from build123d import *

# Parameters (mm, degrees)
SKETCH1_W           = 150.5
SKETCH1_H           = 50
BOSS_EXTRUDE1_DEPTH = 3
SKETCH2_R           = 1.5
SKETCH2_R_2         = 1.25
CUT_EXTRUDE1_DEPTH  = 4
SKETCH4_W           = 74
SKETCH4_H           = 3.5
BOSS_EXTRUDE2_DEPTH = 3
SKETCH5_R           = 1.5
CUT_EXTRUDE3_DEPTH  = 4
SKETCH6_W           = 76.5
SKETCH6_H           = 3
SKETCH6_W_2         = 8
SKETCH6_W_3         = 2
SKETCH6_H_2         = 7
SKETCH6_W_4         = 4
SKETCH6_W_5         = 3
SKETCH6_H_3         = 18
SKETCH6_W_6         = 10
BOSS_EXTRUDE3_DEPTH = 18
SKETCH8_W           = 10
SKETCH8_H           = 3
SKETCH8_H_2         = 2
SKETCH8_W_2         = 42
SKETCH8_W_3         = 3
SKETCH8_H_3         = 15
BOSS_EXTRUDE4_DEPTH = 3
CUT_EXTRUDE4_REACH  = 55.5
SKETCH9_W           = 20
SKETCH9_H           = 10
CUT_EXTRUDE5_REACH  = 152.5
SKETCH10_R          = 1.25
SKETCH11_R          = 1.25
CUT_EXTRUDE6_DEPTH  = 54.5
SKETCH12_R          = 1.25
CUT_EXTRUDE7_DEPTH  = 58
SKETCH13_W          = 10
SKETCH13_H          = 1.5
CUT_EXTRUDE8_DEPTH  = 1.5


with BuildPart() as part:
    # Sketch1 → Boss-Extrude1 (new body)
    with BuildSketch(Plane(origin=(0, 0, 0), x_dir=(1, 0, 0), z_dir=(0, 1, 0))):
        with Locations((-39.87052506, -3.090692124)):
            Rectangle(SKETCH1_W, SKETCH1_H)
    extrude(amount=BOSS_EXTRUDE1_DEPTH)

    # Sketch2 → Cut-Extrude1 (cut, through all)
    with BuildSketch(Plane(origin=(0, 3, 0), x_dir=(1, 0, 0), z_dir=(0, 1, 0))):
        with Locations((-65.12052506, 12.159307876)):
            Circle(SKETCH2_R)
        with Locations((-65.12052506, -18.340692124)):
            Circle(SKETCH2_R)
        with Locations((-34.62052506, -18.340692124)):
            Circle(SKETCH2_R)
        with Locations((-34.62052506, 12.159307876)):
            Circle(SKETCH2_R)
        with Locations((17.87947494, -16.590692124)):
            Circle(SKETCH2_R)
        with Locations((17.87947494, 10.409307876)):
            Circle(SKETCH2_R)
        with Locations((-111.62052506, -19.090692124)):
            Circle(SKETCH2_R)
        with Locations((-111.62052506, 12.909307876)):
            Circle(SKETCH2_R)
        with Locations((-87.62052506, 11.909307876)):
            Circle(SKETCH2_R_2)
        with Locations((-87.62052506, -18.090692124)):
            Circle(SKETCH2_R_2)
        with Locations((-51.62052506, 12.909307876)):
            Circle(SKETCH2_R)
        with Locations((-51.62052506, -19.090692124)):
            Circle(SKETCH2_R)
    extrude(amount=-CUT_EXTRUDE1_DEPTH, mode=Mode.SUBTRACT)

    # Sketch4 → Boss-Extrude2 (add)
    with BuildSketch(Plane(origin=(0, 3, 0), x_dir=(1, 0, 0), z_dir=(0, 1, 0))):
        with Locations((-1.62052506, -29.840692124)):
            Rectangle(SKETCH4_W, SKETCH4_H)
        with Locations((-1.62052506, 23.659307876)):
            Rectangle(SKETCH4_W, SKETCH4_H)
    extrude(amount=-BOSS_EXTRUDE2_DEPTH)

    # Sketch5 → Cut-Extrude3 (cut, through all)
    with BuildSketch(Plane(origin=(0, 3, 0), x_dir=(1, 0, 0), z_dir=(0, 1, 0))):
        with Locations((-34.12052506, 19.409307876)):
            Circle(SKETCH5_R)
        with Locations((-34.12052506, -25.590692124)):
            Circle(SKETCH5_R)
        with Locations((10.87947494, 19.409307876)):
            Circle(SKETCH5_R)
        with Locations((10.87947494, -25.590692124)):
            Circle(SKETCH5_R)
    extrude(amount=-CUT_EXTRUDE3_DEPTH, mode=Mode.SUBTRACT)

    # Sketch6 → Boss-Extrude3 (add)
    with BuildSketch(Plane(origin=(0, 3, 0), x_dir=(1, 0, 0), z_dir=(0, 1, 0))):
        Polygon((35.37947494, 25.409307876), (31.37947494, 25.409307876), (31.37947494, 22.409307876), (32.37947494, 22.409307876), (35.37947494, 22.409307876), align=None)
        with Locations((-76.87052506, -26.590692124)):
            Rectangle(SKETCH6_W, SKETCH6_H)
        with Locations((-76.87052506, 20.409307876)):
            Rectangle(SKETCH6_W, SKETCH6_H)
        with Locations((-34.62052506, 23.909307876)):
            Rectangle(SKETCH6_W_2, SKETCH6_H)
        with Locations((-34.62052506, -30.090692124)):
            Rectangle(SKETCH6_W_2, SKETCH6_H)
        with Locations((-37.62052506, -25.090692124)):
            Rectangle(SKETCH6_W_3, SKETCH6_H_2)
        with Locations((-37.62052506, 18.909307876)):
            Rectangle(SKETCH6_W_3, SKETCH6_H_2)
        with Locations((33.37947494, -30.090692124)):
            Rectangle(SKETCH6_W_4, SKETCH6_H)
        with Locations((33.87947494, -19.590692124)):
            Rectangle(SKETCH6_W_5, SKETCH6_H_3)
        with Locations((33.87947494, 13.409307876)):
            Rectangle(SKETCH6_W_5, SKETCH6_H_3)
        with Locations((16.37947494, -30.090692124)):
            Rectangle(SKETCH6_W_6, SKETCH6_H)
        with Locations((16.37947494, 23.909307876)):
            Rectangle(SKETCH6_W_6, SKETCH6_H)
    extrude(amount=BOSS_EXTRUDE3_DEPTH)

    # Sketch8 → Boss-Extrude4 (add)
    with BuildSketch(Plane(origin=(0, 3, 0), x_dir=(1, 0, 0), z_dir=(0, 1, 0))):
        with Locations((26.37947494, -30.090692124)):
            Rectangle(SKETCH8_W, SKETCH8_H)
        with Locations((26.37947494, 24.409307876)):
            Rectangle(SKETCH8_W, SKETCH8_H_2)
        with Locations((-9.62052506, 23.909307876)):
            Rectangle(SKETCH8_W_2, SKETCH8_H)
        with Locations((-9.62052506, -30.090692124)):
            Rectangle(SKETCH8_W_2, SKETCH8_H)
        with Locations((33.87947494, -3.090692124)):
            Rectangle(SKETCH8_W_3, SKETCH8_H_3)
    extrude(amount=BOSS_EXTRUDE4_DEPTH)

    # Sketch9 → Cut-Extrude4 (cut, up to next)
    with BuildSketch(Plane(origin=(0, 0, -21.909307876), x_dir=(-1, 0, 0), z_dir=(0, 0, -1)), mode=Mode.PRIVATE) as cut_extrude4_sk1:
        with Locations((88.62052506, 13)):
            Rectangle(SKETCH9_W, SKETCH9_H)
    cut_extrude4_tool1 = extrude(cut_extrude4_sk1.sketch, amount=-CUT_EXTRUDE4_REACH, mode=Mode.PRIVATE) & part.part
    add(cut_extrude4_tool1.solids().sort_by_distance((-88.620525, 13, -21.909308))[0], mode=Mode.SUBTRACT)

    # Sketch10 → Cut-Extrude5 (cut, up to next)
    with BuildSketch(Plane(origin=(35.37947494, 0, 0), x_dir=(0, 0, -1), z_dir=(1, 0, 0)), mode=Mode.PRIVATE) as cut_extrude5_sk1:
        with Locations((-21.590692124, 16)):
            Circle(SKETCH10_R)
    cut_extrude5_tool1 = extrude(cut_extrude5_sk1.sketch, amount=-CUT_EXTRUDE5_REACH, mode=Mode.PRIVATE) & part.part
    add(cut_extrude5_tool1.solids().sort_by_distance((35.379475, 16, 21.590692))[0], mode=Mode.SUBTRACT)
    # Sketch10 → Cut-Extrude5 (cut, up to next)
    with BuildSketch(Plane(origin=(35.37947494, 0, 0), x_dir=(0, 0, -1), z_dir=(1, 0, 0)), mode=Mode.PRIVATE) as cut_extrude5_sk2:
        with Locations((15.409307876, 16)):
            Circle(SKETCH10_R)
    cut_extrude5_tool2 = extrude(cut_extrude5_sk2.sketch, amount=-CUT_EXTRUDE5_REACH, mode=Mode.PRIVATE) & part.part
    add(cut_extrude5_tool2.solids().sort_by_distance((35.379475, 16, -15.409308))[0], mode=Mode.SUBTRACT)

    # Sketch11 → Cut-Extrude6 (cut, through all)
    with BuildSketch(Plane(origin=(0, 0, -21.909307876), x_dir=(-1, 0, 0), z_dir=(0, 0, -1))):
        with Locations((43.62052506, 16)):
            Circle(SKETCH11_R)
        with Locations((110.12052506, 16)):
            Circle(SKETCH11_R)
        with Locations((52.62052506, 16)):
            Circle(SKETCH11_R)
        with Locations((101.12052506, 16)):
            Circle(SKETCH11_R)
    extrude(amount=-CUT_EXTRUDE6_DEPTH, mode=Mode.SUBTRACT)

    # Sketch12 → Cut-Extrude7 (cut, through all)
    with BuildSketch(Plane(origin=(0, 0, -25.409307876), x_dir=(-1, 0, 0), z_dir=(0, 0, -1))):
        with Locations((34.62052506, 16)):
            Circle(SKETCH12_R)
    extrude(amount=-CUT_EXTRUDE7_DEPTH, mode=Mode.SUBTRACT)

    # Sketch13 → Cut-Extrude8 (cut)
    with BuildSketch(Plane(origin=(0, 0, 0), x_dir=(-1, 0, 0), z_dir=(0, -1, 0))):
        with Locations((23.62052506, -30.840692124)):
            Rectangle(SKETCH13_W, SKETCH13_H)
        with Locations((23.62052506, 24.659307876)):
            Rectangle(SKETCH13_W, SKETCH13_H)
    extrude(amount=-CUT_EXTRUDE8_DEPTH, mode=Mode.SUBTRACT)


solid = part.part
Input: part model. Units: mm. Frame: model coordinates. A direction names the side the tool comes from. Give positions to 0.01 mm unless a question says otherwise; leave off trailing zeros. Write each loop counter-clockwise with the first axis right and the second up, starting at its lowest first coordinate (ties: lowest second). Pieces come first, ordered by that corner, then holes.
Q1. Pull-direction query (X, two-part tool) for faces 4 (the face through (-30.621, 13, -24)), 5 (the face through (16, 21, -24)); classes: pulls with the +X half, pulls with the -X half, needs draft (parallel to the pull), parting line crosses it, or undercut.
Q2. Material intervals for probe 1 along Z at (x, y) = (-76.5, 10.25); probe 2 along X at (y, z) = (5.5, 26); probe 3 along Z at (x, y) = (-9, 3.5), sorted ascending.
Q3. Section C-C, the plane x = -2.5. Output: boundary loops of the cut face in (y, z), plus the area to 3 significant figures.
Q4. Set-up query: faces 1 (the face through (-10, 6, 30)), 2 (the face through (26, 4, -23.409)), 3 (the face through (-77, 10, 28.091)). Return all of +Z, -Z, +X, -X, +Y, -Y with unobstructed straight access to the full face (end or side cutting, diameter ignored); none if empty.
Q5. Section A-A, the plane x = -26. Output: boundary loops of the cut face in (y, z).
Q6. First-contact query: P1, Ø1, axis at y = 7, z = 30, coming from the -X side; P2, Ø1.2, axis at x = -24.5, y = 0.5, coming from the -Z side; P3, Ø2.5, axis at x = 17.88, z = -10.41, coming from the -Y side; P4, Ø4, axis at x = 10.88, z = 25.59, coming from the +Y side. Flat tips, straight axial feed; report the tip coordinate or a pass-through.
Q7. Section B-B, the plane z = 0. Output: boundary loops of the cut face in (x, y).
Q8. Section D-D, the plane z = -7. Output: boundary loops of the cut face in (x, y).
Filled in:
1. face 4: undercut
1. face 5: needs draft
2. probe 1: z = -21.91 to -18.91, 25.09 to 28.09
2. probe 2: x = -115.12 to -36.62, 32.38 to 35.38
2. probe 3: z = -25.41 to -22.41, 28.59 to 31.59
3. outline: (0, -25.41) - (6, -25.41) - (6, -22.41) - (3, -22.41) - (3, 28.59) - (6, 28.59) - (6, 31.59) - (0, 31.59) - close
3. area: 189 mm2
4. face 1: +Z, -Z, +Y
4. face 2: +Y
4. face 3: +Z, -X, +Y, -Y
5. outline: (0, -23.91) - (1.5, -23.91) - (1.5, -25.41) - (6, -25.41) - (6, -22.41) - (3, -22.41) - (3, 28.59) - (6, 28.59) - (6, 31.59) - (1.5, 31.59) - (1.5, 30.09) - (0, 30.09) - close
6. P1: stops at x = -38.62
6. P2: stops at z = -23.91
6. P3: passes through
6. P4: stops at y = 3
7. outline: (-115.12, 0) - (35.38, 0) - (35.38, 6) - (32.38, 6) - (32.38, 3) - (-115.12, 3) - close
8. outline: (-115.12, 0) - (35.38, 0) - (35.38, 21) - (32.38, 21) - (32.38, 3) - (-115.12, 3) - close
